Autodesk Inventor part; units mm, degrees
ref_plane "YZ Plane" through (0, 0, 0) normal (1, 0, 0) x (0, 1, 0)
ref_plane "XZ Plane" through (0, 0, 0) normal (0, 1, 0) x (-1, 0, 0)
ref_plane "XY Plane" through (0, 0, 0) normal (0, 0, 1) x (1, 0, 0)
sketch "Sketch1" plane through (0, 0, 0) normal (0, 1, 0) x (-1, 0, 0)
  line L0 (0, 0) -> (-61, 0)
  line L1 (-61, 0) -> (-61, -30)
  line L2 (-61, -30) -> (0, -30)
  line L3 (0, -30) -> (0, 0)
  dimension "d0" = 30
  dimension "d1" = 61
extrude "Extrusion1" add sketch "Sketch1" along normal blind 3
fillet "Fillet1" radius 1 4 edges at (0, 1.5, 0) (61, 1.5, 0) (61, 1.5, -30) (0, 1.5, -30)
sketch "Sketch4" plane through (0, 0, 0) normal (0, -1, 0) x (1, 0, 0)
  line L0 (2.125, -2) -> (5.875, -2)
  line L1 (5.875, -2) -> (5.875, 0)
  line L2 (5.875, 0) -> (2.125, 0)
  line L3 (2.125, 0) -> (2.125, -2)
  line L4 (55.125, -2) -> (58.875, -2)
  line L5 (58.875, -2) -> (58.875, 0)
  line L6 (58.875, 0) -> (55.125, 0)
  line L7 (55.125, 0) -> (55.125, -2)
  line L8 (0, -29) -> (0, -1)
  line L9 (1, 0) -> (60, 0)
  line L10 (61, -1) -> (61, -29)
  point P0 (0, 0)
  dimension "d31" = 3.75
  dimension "d32" = 3.75
  dimension "d33" = 2
  dimension "d34" = 2
  dimension "d35" = 5.875
  dimension "d36" = 0
  dimension "d37" = 0
  dimension "d38" = 5.875
extrude "Extrusion3" add sketch "Sketch4" along normal blind 1
sketch "Sketch2" plane through (0, 3, 0) normal (0, 1, 0) x (1, 0, 0)
  circle A0 centre (4, 8) radius 1
  line L0 (0, 0) -> (61, 0)
  line L1 (0, 30) -> (0, 0)
  circle A1 centre (57, 8) radius 1
  line L2 (61, 0) -> (61, 30)
  circle A2 centre (4, 26) radius 1
  circle A3 centre (57, 26) radius 1
  line L3 (61, 30) -> (0, 30)
  dimension "d4" = 8
  dimension "d5" = 4
  dimension "d6" = 2
  dimension "d7" = 2
  dimension "d8" = 4
  dimension "d9" = 8
  dimension "d10" = 2
  dimension "d11" = 2
  dimension "d12" = 4
  dimension "d13" = 4
  dimension "d14" = 4
  dimension "d15" = 4
hole "Hole1" at (4, 3, -26) at (4, 3, -8) at (57, 3, -8) at (57, 3, -26) direction (0, -1, 0) diameter 2.1 end through all countersink diameter 3.75 countersink angle 90
sketch "Sketch6" plane through (0, 0, 0) normal (0, -1, 0) x (1, 0, 0)
  line L0 (16.5, -10) -> (27.5, -10)
  line L1 (27.5, -10) -> (27.5, 0)
  line L2 (27.5, 0) -> (16.5, 0)
  line L3 (16.5, 0) -> (16.5, -10)
  line L4 (1, 0) -> (60, 0)
  line L5 (0, -29) -> (0, -1)
  line L6 (16.5, -30) -> (27.5, -30)
  line L7 (27.5, -30) -> (27.5, -20)
  line L8 (27.5, -20) -> (16.5, -20)
  line L9 (16.5, -20) -> (16.5, -30)
  line L10 (60, -30) -> (1, -30)
  point P0 (0, 0)
  dimension "d48" = 16.5
  dimension "d49" = 11
  dimension "d50" = 10
  dimension "d51" = 0
  dimension "d52" = 10
  dimension "d53" = 16.5
  dimension "d55" = 11
  dimension "d56" = 0
extrude "Extrusion4" cut sketch "Sketch6" against normal blind 1
equation "\"d52\" = d50"
equation "\"d53\" = d48"
properties part number "Link Adapter Top"
CAD build for the part. Positions are in the model's coordinates, mm. A direction names the side the tool comes from. Round coordinates to 2 decimals unless told otherwise and drop trailing zeros. Write each loop counter-clockwise with the first axis right and the second up, starting at its lowest first coordinate (ties: lowest second). Pieces come first, ordered by that corner, then holes.
(1) 3-axis set-ups, long thin cutter, end or side, ignore diameter. For faces 1 (the face through (22, 1, -25)), 2 (the face through (22, 1, -5)), 3 (the face through (57, -1, -1)): which of +Z, -Z, +X, -X, +Y, -Y reach the whole face in a straight line?
(2) Drop flat-ended pins along their axis: P1, Ø0.8, axis at x = 57.5, y = -0.5, coming from the -Z side; P2, Ø8, axis at x = 53.5, z = -20.5, coming from the -Y side; P3, Ø0.8, axis at x = 20.5, y = 0.5, coming from the -Z side. Give the stop position or say it passes through.
(3) Probe line 1 along X through (y, z) = (0.85, -8); line 2 along X through (y, z) = (1.1, -8); line 3 along Z through (x, y) = (4, 1.2). List the from-to ranges inside material, lowest first.
(4) Slice it at A-A, the plane x = 4. Write the cut outline in (y, z) (3 decimals).
(5) Slice it at B-B, the plane z = -26. Write the cut outline in (x, y) (3 decimals), and give its area (3 significant figures).
(6) Slice it at C-C, the plane x = 22. Write the cut outline in (y, z), and give its area (3 significant figures).
(7) Slice it at D-D, the plane z = -18. Write the cut outline in (x, y), and give its area (3 significant figures).
(8) Mould opens along Z. For faces 4 (the face through (58.025, 1.072, -8.228)), 5 (the face through (31, 3, -15)), 6 (the face through (31, 1, -30)), 7 (the face through (2.96, 1.07, -8.14)) say: pulls with the +Z half, pulls with the -Z half, needs draft (parallel to the pull), parting line crosses it, or undercut.
From the geometry:
1. face 1: -Z, -Y
1. face 2: +Z, -Y
1. face 3: +Z, -Z, +X, -X, -Y
2. P1: stops at z = -2
2. P2: stops at y = 0
2. P3: stops at z = -20
3. line 1: x = 0 to 2.95, 5.05 to 16.5, 27.5 to 55.95, 58.05 to 61
3. line 2: x = 0 to 2.95, 5.05 to 55.95, 58.05 to 61
3. line 3: z = -30 to -27.05, -24.95 to -9.05, -6.95 to 0
4. outline: (-1, -2) - (0, -2) - (0, -6.95) - (2.175, -6.95) - (3, -6.125) - (3, 0) - (-1, 0) - close; (0, -30) - (3, -30) - (3, -27.875) - (2.175, -27.05) - (0, -27.05) - close; (0, -24.95) - (2.175, -24.95) - (3, -24.125) - (3, -9.875) - (2.175, -9.05) - (0, -9.05) - close
5. outline: (0, 0) - (2.95, 0) - (2.95, 2.175) - (2.125, 3) - (0, 3) - close; (5.05, 0) - (16.5, 0) - (16.5, 1) - (27.5, 1) - (27.5, 0) - (55.95, 0) - (55.95, 2.175) - (55.125, 3) - (5.875, 3) - (5.05, 2.175) - close; (58.05, 0) - (61, 0) - (61, 3) - (58.875, 3) - (58.05, 2.175) - close
5. area: 158 mm2
6. outline: (0, -20) - (1, -20) - (1, -30) - (3, -30) - (3, 0) - (1, 0) - (1, -10) - (0, -10) - close
6. area: 70.0 mm2
7. outline: (0, 0) - (61, 0) - (61, 3) - (0, 3) - close
7. area: 183 mm2
8. face 4: undercut
8. face 5: needs draft
8. face 6: pulls with the -Z half
8. face 7: undercut
